Geometry: final body of the model. Coordinates: model frame, mm. Face numbers are marked on the shaded views. A direction names the side the tool comes from. Give positions to 0.01 mm unless a question says otherwise; leave off trailing zeros. Write each loop counter-clockwise with the first axis right and the second up, starting at its lowest first coordinate (ties: lowest second). Pieces come first, ordered by that corner, then holes. Notation, with made-up numbers: M 24,16.25 L 70,16.25 A16 cw 70,33.25 Z; hole C 7,46.5 d6. An arc over 180 degrees is marked long. Use a Markdown table: item, result. Add a question column.
1) Section C-C on x = -12.5. Return the cut outline in (y, z).
2) Section A-A on z = 0. Return the cut outline in (x, y).
3) Section D-D on y = 16. Return the cut outline in (x, z).
4) Draft query along X for the marked faces 1, 2, 3 and 4. Return one class per face: +X half, -X half, draft (parallel to the pull), parting line (faces both ways), or undercut.
5) Line query: line 1 (X direction, y = 19, z = -1); line 2 (Y direction, x = 3.5, z = 4.5); line 3 (X direction, y = 50, z = 2). Output: solid intervals per line, ascending.
6) Section B-B on y = 44. Return the cut outline in (x, z).
7) Pin query (flat end, axial travel): pin 1 (12 mm diameter, centred on x = -20, z = 6, fed in from -Y); pin 2 (1.5 mm diameter, centred on y = 36, z = -15, fed in from -X); pin 3 (17 mm diameter, centred on x = -34.5, z = 0.5, fed in from -Y); pin 4 (7.5 mm diameter, centred on y = 40.5, z = -4, fed in from +X). Return the tip coordinate at first contact, or that it passes through.
8) Set-up query: the marked faces 5, 6, 7 and 8. Return all of +Z, -Z, +X, -X, +Y, -Y with unobstructed straight access to the full face (end or side cutting, diameter ignored); none if empty.
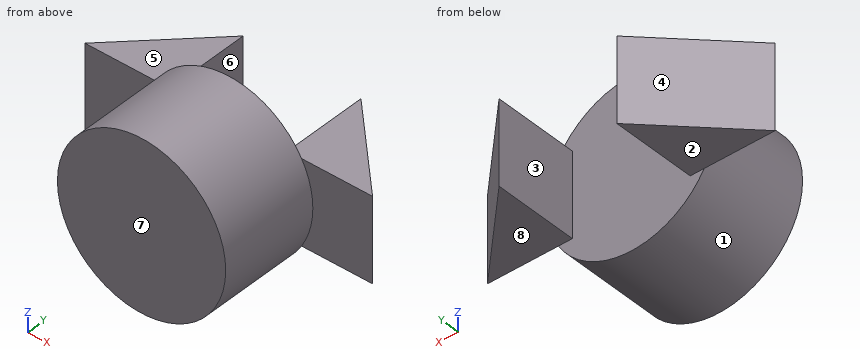
```python
from build123d import *

# Parameters (mm, degrees)
SKETCH_1_R          = 25
EXTRUDE_1_DEPTH     = 30
EXTRUDE_2_DEPTH     = 12.5
CUT_EXTRUDE_1_DEPTH = 19


with BuildPart() as part:
    # 草图1 → 凸台-拉伸1 (new body)
    with BuildSketch(Plane(origin=(0, 0, 0), x_dir=(1, 0, 0), z_dir=(0, 1, 0))):
        Circle(SKETCH_1_R)
    extrude(amount=EXTRUDE_1_DEPTH)

    # 草图3 → 凸台-拉伸2 (add, symmetric)
    with BuildSketch(Plane.XY):
        Polygon((42.744510846, 30), (-42.744510846, 30), (0, 72.744510846), align=None)
    extrude(amount=EXTRUDE_2_DEPTH, both=True)

    # 草图4 → 切除-拉伸1 (cut, symmetric)
    with BuildSketch(Plane.XY):
        Polygon((17.500255974, 30), (-17.500255974, 30), (-17.500255974, 55.244254872), (0, 72.744510846), (17.500255974, 55.244254872), align=None)
    extrude(amount=CUT_EXTRUDE_1_DEPTH, both=True, mode=Mode.SUBTRACT)


solid = part.part
```
Found:
| question | item | result |
|---|---|---|
| 1 | outline | M 0,-21.65 L 30,-21.65 L 30,21.65 L 0,21.65 Z |
| 2 | outline | M -42.74,30 L -25,30 L -25,0 L 25,0 L 25,30 L 42.74,30 L 17.5,55.24 L 17.5,30 L -17.5,30 L -17.5,55.24 Z |
| 3 | outline | C 0,0 d50 |
| 4 | face 1 | parting line |
| 4 | face 2 | draft |
| 4 | face 3 | undercut |
| 4 | face 4 | -X half |
| 5 | line 1 | -24.98 to 24.98 |
| 5 | line 2 | 0 to 30 |
| 5 | line 3 | -22.74 to -17.5, 17.5 to 22.74 |
| 6 | outline | M -28.74,-12.5 L -17.5,-12.5 L -17.5,12.5 L -28.74,12.5 Z; M 17.5,-12.5 L 28.74,-12.5 L 28.74,12.5 L 17.5,12.5 Z |
| 7 | pin 1 | y = 0 |
| 7 | pin 2 | through |
| 7 | pin 3 | y = 30 |
| 7 | pin 4 | x = 35.99 |
| 8 | face 5 | +Z, +X, -X, +Y |
| 8 | face 6 | +Z, -Z, +Y |
| 8 | face 7 | +Z, -Z, +X, -X, -Y |
| 8 | face 8 | -Z, +X, -X, +Y |
